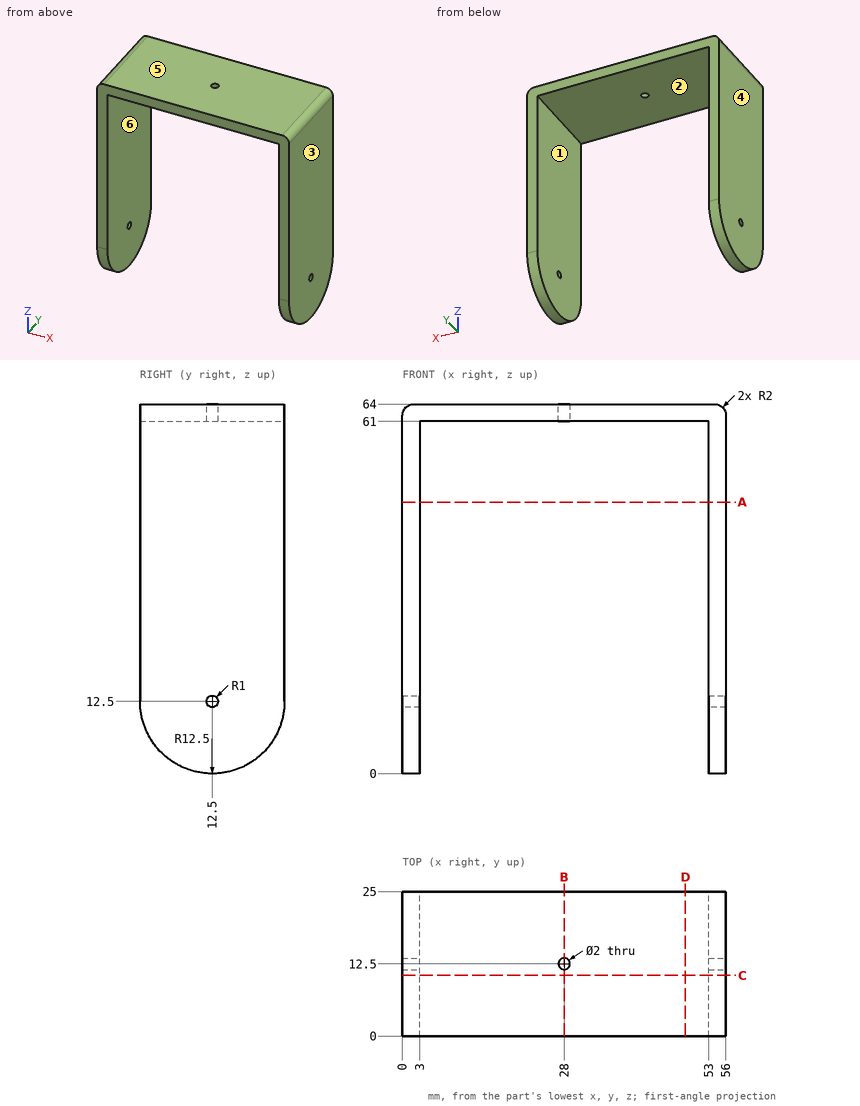
Here's the drawing with two shaded views (mm, measured from the low corner). I have some questions. A direction names the side the tool comes from. Coordinates: 2 decimals unless noted, no trailing zeros. Write each loop counter-clockwise with the first axis right and the second up, starting at its lowest first coordinate (ties: lowest second). Pieces come first, ordered by that corner, then holes.
Item 1: I want a section at D-D on x = 49. Write out the boundary of the cut face in (y, z).
Item 2: If I drill on line 1 (X direction, y = 9, z = 44); line 2 (Y direction, x = 28, z = 63.05); line 3 (Z direction, x = 10.5, y = 13), over which ranges is the centre line in solid material (lowest first)?
Item 3: If we mould it in two halves opening along X, with no side actions, what happens to the marked faces 1, 2, 3 and 4? For each: +X half, -X half, draft (parallel to the pull), parting line (faces both ways), or undercut.
Item 4: I want a section at B-B on x = 28. Write out the boundary of the cut face in (y, z).
Item 5: Will this pin go through, and if not, where does the flat tip stop? pin 1 (1.5 mm diameter, centred on x = 29, y = 5, fed in from -Z).
Item 6: I want a section at A-A on z = 47. Write out the boundary of the cut face in (x, y).
Item 7: On a 3-axis mill with a long thin cutter (end or side, diameter ignored), from which of +Z, -Z, +X, -X, +Y, -Y can I reach the whole of each face in a straight line? I mean the marked faces 5 and 6. Say none if no direction works.
Item 8: I want a section at C-C on y = 10.5. Write out the boundary of the cut face in (x, z).
Findings below:
1. outline: (0, 61) - (25, 61) - (25, 64) - (0, 64) - close
2. line 1: x = 0 to 3, 53 to 56
2. line 2: y = 0 to 11.5, 13.5 to 25
2. line 3: z = 61 to 64
3. face 1: undercut
3. face 2: undercut
3. face 3: +X half
3. face 4: -X half
4. outline: (0, 61) - (11.5, 61) - (11.5, 64) - (0, 64) - close; (13.5, 61) - (25, 61) - (25, 64) - (13.5, 64) - close
5. pin 1: stops at z = 61
6. outline: (0, 0) - (3, 0) - (3, 25) - (0, 25) - close; (53, 0) - (56, 0) - (56, 25) - (53, 25) - close
7. face 5: +Z, +X, -X, +Y, -Y
7. face 6: -Z, +Y, -Y
8. outline: (0, 0.16) - (3, 0.16) - (3, 61) - (53, 61) - (53, 0.16) - (56, 0.16) - (56, 62) arc R2 ccw to (54, 64) - (2, 64) arc R2 ccw to (0, 62) - close
